Read the model definition and answer for the solid it produces. Units are mm, in the model's axes. A direction names the side the tool comes from. Coordinates: 2 decimals unless noted, no trailing zeros. Order: outer loops, then holes, each group sorted by start corner. A loop starts at its lowest first (then second) coordinate and runs counter-clockwise, first axis right, second up. Notation, with made-up numbers: M 12.5,23.25 L 45.5,23.25 A22 ccw 45.5,31.25 Z; hole C 21,68.25 d11. An arc over 180 degrees is marked long. Use a Markdown table: item, result. Add a question column.
1) Each of these flat-tipped pins is pushed along its axis until it touches: pin 1 Ø4 at (y, z) = (-7, 9.5) entering from -X; pin 2 Ø4.5 at (y, z) = (-10.5, 70) entering from +X; pin 3 Ø12 at (x, y) = (28.5, -20) entering from +Z. Where does it stop, or does it pass through?
2) The mould has two halves that part along Y. Classify faces 4 (the face through (160, -8, 9)), 5 (the face through (132, -13, 20)), 6 (the face through (16, -27, 43)): released by +Y, released by -Y, zero draft, split by the parting line, or undercut.
3) Find section C-C on x = 110. Write down the section's boundary in (y, z).
4) For faces 1 (the face through (76.25, -14, 14)), 2 (the face through (13, -14.5, 67.6)), 3 (the face through (165, -16, 75)), determine the directions among +Z, -Z, +X, -X, +Y, -Y from which every point of the face is accessible in a straight line to the end or side of a thin tool.
5) Find section A-A on x = 90. Write down the section's boundary in (y, z).
6) Find section B-B on z = 22.5. Write down the section's boundary in (x, y), plus the area to 3 significant figures.
7) Find the intervals of material crossed by probe 1 along Y at (x, z) = (165, 69); probe 2 along X at (y, z) = (-13.5, 2.25); probe 3 along Y at (x, z) = (168, 8), in increasing order. Write a range as [from, to].
from build123d import *

# Parameters (mm, degrees)
F0_W         = 180
F0_H         = 90
F1_DEPTH     = 27
F2_W         = 140
F2_H         = 70
F3_DEPTH     = 27.001
F4_W         = 10
F4_H         = 10
F5_DEPTH     = 27.001
F6_R         = 2.5
F7_DEPTH     = 80
F9_DEPTH     = 180.001
F11_R        = 2.5
F12_DEPTH    = 20
F10_R        = 2.5
F13_DEPTH    = 20
F14_T1_DEPTH = 155
F15_W        = 27.5
F15_H        = 10
F16_DEPTH    = 27.0010001
F18_SIZE     = 1
F19_R        = 2.5
F20_DEPTH    = 90.0010001


# Not quite as in the source:
# - a fillet or chamfer that OpenCascade refuses, or shapes differently, is made with other operations: its cross-section is extruded or revolved along the edge and cut away or added


with BuildPart() as f1:
    # F0 (on Front) → F1 (new body)
    with BuildSketch(Plane.XZ):
        with Locations((90, 45)):
            Rectangle(F0_W, F0_H)
    extrude(amount=F1_DEPTH)

    # F2 (on Front) → F3 (cut, through all)
    with BuildSketch(Plane.XZ):
        with Locations((90, 55)):
            Rectangle(F2_W, F2_H)
    extrude(amount=F3_DEPTH, mode=Mode.SUBTRACT)

    # F4 (on Front) → F5 (cut, through all)
    with BuildSketch(Plane.XZ):
        with Locations((165, 80)):
            Rectangle(F4_W, F4_H)
        with Locations((165, 55)):
            Rectangle(F4_W, F4_H)
        with Locations((165, 30)):
            Rectangle(F4_W, F4_H)
        with Locations((15, 30)):
            Rectangle(F4_W, F4_H)
        with Locations((15, 55)):
            Rectangle(F4_W, F4_H)
        with Locations((15, 80)):
            Rectangle(F4_W, F4_H)
    extrude(amount=F5_DEPTH, mode=Mode.SUBTRACT)

    # F6 (on face) → F7 (cut)
    with BuildSketch(Plane.XY.offset(90)):
        with Locations((165, -13)):
            Circle(F6_R)
        with Locations((15, -13)):
            Circle(F6_R)
    extrude(amount=-F7_DEPTH, mode=Mode.SUBTRACT)

    # F8 (on Right) → F9 (cut, through all)
    with BuildSketch(Plane.YZ):
        with BuildLine():
            Line((-13, 77.5), (-13, 82.5))
            ThreePointArc((-13, 82.5), (-15.5, 80), (-13, 77.5))
        make_face()
        with BuildLine():
            ThreePointArc((-13, 77.5), (-11.232233047, 78.232233047), (-10.5, 80))
            ThreePointArc((-10.5, 80), (-11.232233047, 81.767766953), (-13, 82.5))
            Line((-13, 82.5), (-13, 77.5))
        make_face()
        with BuildLine():
            Line((-13, 52.5), (-13, 57.5))
            ThreePointArc((-13, 57.5), (-15.5, 55), (-13, 52.5))
        make_face()
        with BuildLine():
            ThreePointArc((-10.5, 55), (-11.232233047, 56.767766953), (-13, 57.5))
            Line((-13, 57.5), (-13, 52.5))
            ThreePointArc((-13, 52.5), (-11.232233047, 53.232233047), (-10.5, 55))
        make_face()
        with BuildLine():
            Line((-13, 27.5), (-13, 32.5))
            ThreePointArc((-13, 32.5), (-15.5, 30), (-13, 27.5))
        make_face()
        with BuildLine():
            ThreePointArc((-10.5, 30), (-11.232233047, 31.767766953), (-13, 32.5))
            Line((-13, 32.5), (-13, 27.5))
            ThreePointArc((-13, 27.5), (-11.232233047, 28.232233047), (-10.5, 30))
        make_face()
    extrude(amount=F9_DEPTH, mode=Mode.SUBTRACT)

    # F11 (on face) → F12 (cut)
    with BuildSketch(Plane.YZ.offset(180)):
        with Locations((-8, 8.5)):
            Circle(F11_R)
        with Locations((-18, 8.5)):
            Circle(F11_R)
    extrude(amount=-F12_DEPTH, mode=Mode.SUBTRACT)

    # F10 (on Right) → F13 (cut)
    with BuildSketch(Plane.YZ):
        with Locations((-8, 8.5)):
            Circle(F10_R)
        with Locations((-18, 8.5)):
            Circle(F10_R)
    extrude(amount=F13_DEPTH, mode=Mode.SUBTRACT)

    # F14: fillet of radius 13 on 4 edges, made by hand

    # F14_s2 → F14_t1 (cut)
    with BuildSketch(Plane.XY.offset(-32.5)):
        with BuildLine():
            ThreePointArc((0, -13), (3.8076118446, -3.8076118446), (13, 0))
            Line((13, 0), (0, 0))
            Line((0, 0), (0, -13))
        make_face()
        with BuildLine():
            ThreePointArc((0, -14), (3.8076118446, -23.1923881554), (13, -27))
            Line((13, -27), (0, -27))
            Line((0, -27), (0, -14))
        make_face()
        with BuildLine():
            ThreePointArc((167, -27), (176.1923881554, -23.1923881554), (180, -14))
            Line((180, -14), (180, -27))
            Line((180, -27), (167, -27))
        make_face()
        with BuildLine():
            ThreePointArc((167, 0), (176.1923881554, -3.8076118446), (180, -13))
            Line((180, -13), (180, 0))
            Line((180, 0), (167, 0))
        make_face()
    extrude(amount=F14_T1_DEPTH, mode=Mode.SUBTRACT)

    # F15 (on face) → F16 (cut, through all)
    with BuildSketch(Plane.XZ.offset(27)):
        with Locations((90, 15)):
            Rectangle(F15_W, F15_H)
    extrude(amount=-F16_DEPTH, mode=Mode.SUBTRACT)

    # F18
    f18_edges = [f1.edges().sort_by_distance(p)[0] for p in [
        (103.75, -13.5, 20),
        (76.25, -13.5, 20),
    ]]
    chamfer(f18_edges, length=F18_SIZE)

    # F19 (on face) → F20 (cut, through all)
    with BuildSketch(Plane(origin=(0, 0, 0), x_dir=(1, 0, 0), z_dir=(0, 0, -1))):
        with Locations((90, 13.5)):
            Circle(F19_R)
    extrude(amount=-F20_DEPTH, mode=Mode.SUBTRACT)


solid = f1.part
Check result:
| question | item | result |
|---|---|---|
| 1 | pin 1 | stops at x = 0.86 |
| 1 | pin 2 | stops at x = 180 |
| 1 | pin 3 | stops at z = 20 |
| 2 | face 4 | undercut |
| 2 | face 5 | zero draft |
| 2 | face 6 | released by -Y |
| 3 | outline | M -27,0 L 0,0 L 0,20 L -27,20 Z |
| 4 | face 1 | +Z, +Y, -Y |
| 4 | face 2 | +Z |
| 4 | face 3 | +Y, -Y |
| 5 | outline | M -27,0 L -16,0 L -16,10 L -27,10 Z; M -11,0 L 0,0 L 0,10 L -11,10 Z |
| 6 | outline | M 0,-14 A13 ccw 13,-27 L 20,-27 L 20,0 L 13,0 A13 ccw 0,-13 Z; M 160,-27 L 167,-27 A13 ccw 180,-14 L 180,-13 A13 ccw 167,0 L 160,0 Z; hole C 15,-13 d5; hole C 165,-13 d5 |
| 6 | area | 896 mm2 |
| 7 | probe 1 | y = [-27, -15.5], [-10.5, 0] |
| 7 | probe 2 | x = [0, 87.5], [92.5, 180] |
| 7 | probe 3 | y = [-26.96, -20.45], [-15.55, -10.45], [-5.55, -0.04] |
